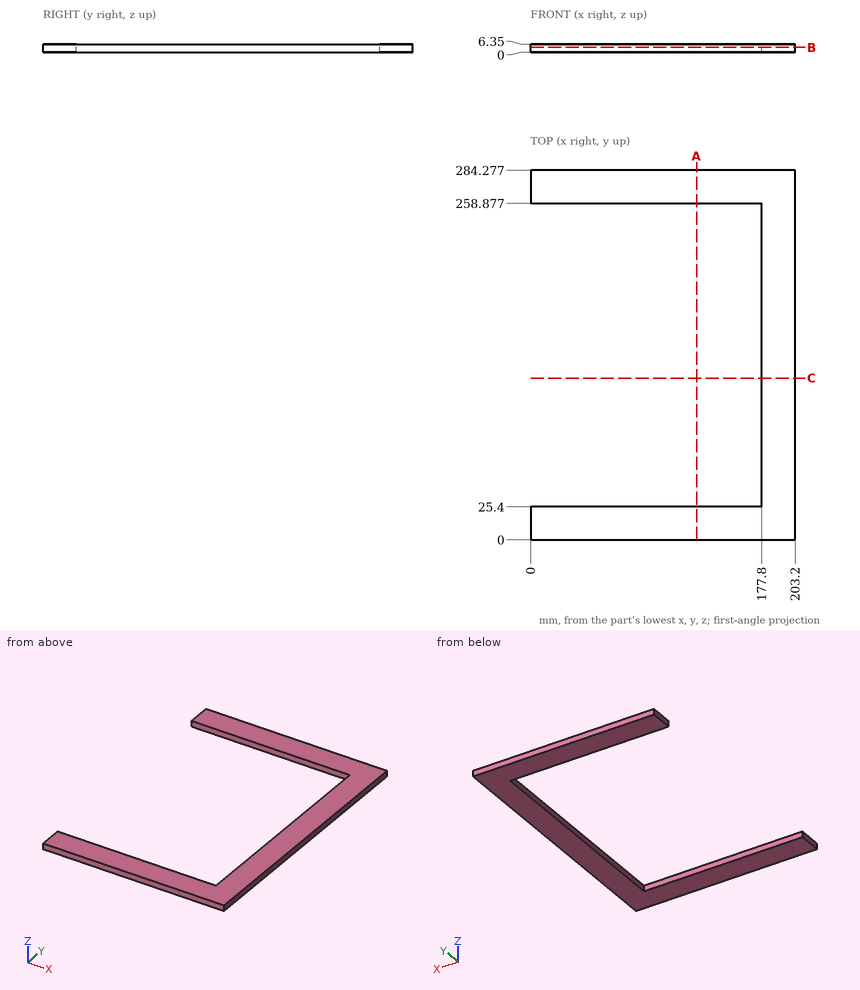
For this review, use the dimensioned drawing (mm, ordinates from the lowest corner) and the shaded views. Round coordinates to 2 decimals unless told otherwise and drop trailing zeros. Write each loop counter-clockwise with the first axis right and the second up, starting at its lowest first coordinate (ties: lowest second). Pieces come first, ordered by that corner, then holes. Notation, with made-up numbers: (-30, -1.75) -> (-12, -1.75) arc R23 cw to (-12, 11.25) -> close; hole circle Ø3 at (49, -12.5). An arc over 180 degrees is marked (long way). One line per item, written item: value. Start each with the question number.
Q1. Insertion check: P1, Ø3, axis at y = 100.5, z = 4, coming from the -X side. The pin has a flat end and moves straight along its axis. Give the tip position at first contact, or say it passes through.
Q2. Add section B-B (z = 3.75). Give the boundary of the cut face in (x, y), then the cut area to 3 significant figures.
Q3. To check wall thickness, follow probe 1 along Y at (x, z) = (90, 5.5); probe 2 along X at (y, z) = (219, 4.75). State the ranges of each line that lie inside material, in increasing order.
Q4. Add section C-C (y = 124.5). Give the boundary of the cut face in (x, z), then the cut area to 3 significant figures.
Q5. Add section A-A (x = 127.5). Give the boundary of the cut face in (y, z).
Response:
1. P1: stops at x = 177.8
2. outline: (0, 0) -> (203.2, 0) -> (203.2, 284.28) -> (0, 284.28) -> (0, 258.88) -> (177.8, 258.88) -> (177.8, 25.4) -> (0, 25.4) -> close
2. area: 16,300 mm^2
3. probe 1: y = 0 to 25.4, 258.88 to 284.28
3. probe 2: x = 177.8 to 203.2
4. outline: (177.8, 0) -> (203.2, 0) -> (203.2, 6.35) -> (177.8, 6.35) -> close
4. area: 161 mm^2
5. outline: (0, 0) -> (25.4, 0) -> (25.4, 6.35) -> (0, 6.35) -> close; (258.88, 0) -> (284.28, 0) -> (284.28, 6.35) -> (258.88, 6.35) -> close
